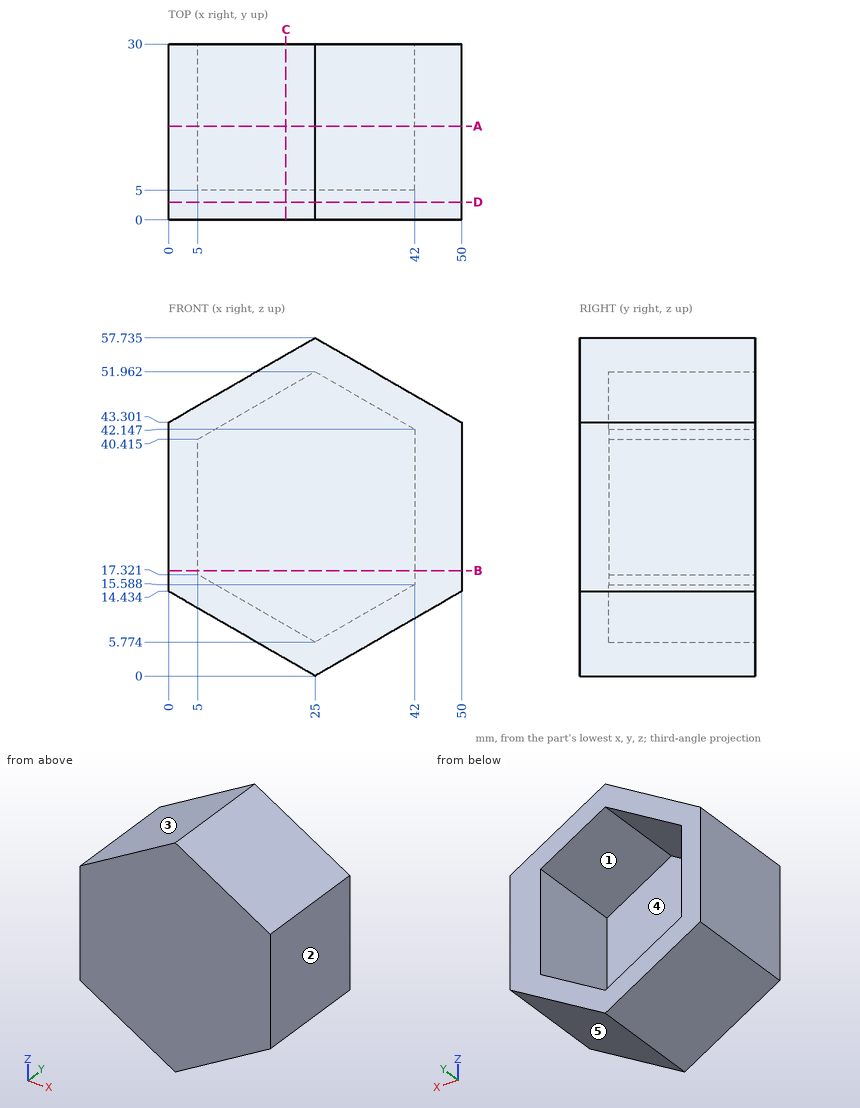
Could you check a few things on this drawing? It's one solid part, dimensions in mm from its lowest x, y, z. A direction names the side the tool comes from. Give positions to 0.01 mm unless a question says otherwise; leave off trailing zeros. Order: outer loops, then holes, each group sorted by start corner. A loop starts at its lowest first (then second) coordinate and runs counter-clockwise, first axis right, second up. Notation, with made-up numbers: (-22, 79) -> (24, 79) arc R35 ccw to (24, 116) -> close; hole circle Ø10 at (-22.75, 22). An arc over 180 degrees is marked (long way). Answer in a Markdown table with one row per item. Add a question column.
Item 1: Imagine slicing it at B-B (z = 18). List the corners of the cut face in (x, y) for me.
Item 2: Please list where these lines run through material, in increasing order: probe 1 along X at (y, z) = (11.25, 32); probe 2 along Y at (x, z) = (13.5, 12.5); probe 3 along Z at (x, y) = (23.5, 28.75) (1 decimal).
Item 3: Imagine slicing it at A-A (y = 16). List the corners of the cut face in (x, z) for me (1 decimal), and give its area (3 significant figures).
Item 4: For the marked faces 1 and 2, which set-ups out of +Z, -Z, +X, -X, +Y, -Y let a thin tool reach every point of the face, with its end or its side?
Item 5: Imagine slicing it at C-C (x = 20). List the corners of the cut face in (y, z) for me (1 decimal).
Item 6: Imagine slicing it at D-D (y = 3). List the corners of the cut face in (x, z) for me (1 decimal), and give its area (4 significant figures).
Item 7: We'd pull the mould along Z, two halves only. Please class the marked faces 3, 4 and 5: pulls with the +Z half, pulls with the -Z half, needs draft (parallel to the pull), parting line crosses it, or undercut.
Item 8: I'm going to push flat-ended pins straight in: P1, Ø4, axis at x = 44.5, y = 25, coming from the +Z side; P2, Ø1.5, axis at x = 33, y = 19, coming from the +Z side; P3, Ø18.5, axis at x = 30, z = 25, coming from the +Y side. Where does each tip first touch, or does it pass through?
Result:
| question | item | result |
|---|---|---|
| 1 | outline | (0, 0) -> (50, 0) -> (50, 30) -> (42, 30) -> (42, 5) -> (5, 5) -> (5, 30) -> (0, 30) -> close |
| 2 | probe 1 | 0 to 5, 42 to 50 |
| 2 | probe 2 | 0 to 5 |
| 2 | probe 3 | 0.9 to 6.6, 51.1 to 56.9 |
| 3 | outline | (0, 14.4) -> (25, 0) -> (50, 14.4) -> (50, 43.3) -> (25, 57.7) -> (0, 43.3) -> close; hole (5, 17.3) -> (25, 5.8) -> (42, 15.6) -> (42, 42.1) -> (25, 52) -> (5, 40.4) -> close |
| 3 | area | 854 mm2 |
| 4 | face 1 | +Y |
| 4 | face 2 | +Z, -Z, +X, +Y, -Y |
| 5 | outline | (0, 2.9) -> (30, 2.9) -> (30, 8.7) -> (5, 8.7) -> (5, 49.1) -> (30, 49.1) -> (30, 54.8) -> (0, 54.8) -> close |
| 6 | outline | (0, 14.4) -> (25, 0) -> (50, 14.4) -> (50, 43.3) -> (25, 57.7) -> (0, 43.3) -> close |
| 6 | area | 2,165 mm2 |
| 7 | face 3 | pulls with the +Z half |
| 7 | face 4 | undercut |
| 7 | face 5 | pulls with the -Z half |
| 8 | P1 | z = 47.63 |
| 8 | P2 | z = 53.55 |
| 8 | P3 | y = 5 |
